from build123d import *

# Parameters (mm, degrees)
CROQUIS1_W              = 633.04
CROQUIS1_H              = 80
CROQUIS1_R              = 4.7625
SALIENTE_EXTRUIR1_DEPTH = 10
CROQUIS2_W              = 633.04
CROQUIS2_H              = 10
SALIENTE_EXTRUIR2_DEPTH = 70
CROQUIS3_R              = 4.7625
CROQUIS3_R_2            = 4.765
CORTAR_EXTRUIR1_DEPTH   = 642.903140357
CORTAR_EXTRUIR2_DEPTH   = 15
CORTAR_EXTRUIR3_DEPTH   = 15


with BuildPart() as part:
    # Croquis1 → Saliente-Extruir1 (new body)
    with BuildSketch(Plane.XY):
        with Locations((316.52, 40)):
            Rectangle(CROQUIS1_W, CROQUIS1_H)
        with Locations((30, 40)):
            Circle(CROQUIS1_R, mode=Mode.SUBTRACT)
        with Locations((603.04, 40)):
            Circle(CROQUIS1_R, mode=Mode.SUBTRACT)
    extrude(amount=SALIENTE_EXTRUIR1_DEPTH)

    # Croquis2 → Saliente-Extruir2 (add)
    with BuildSketch(Plane.XY.offset(10)):
        with Locations((316.52, 75)):
            Rectangle(CROQUIS2_W, CROQUIS2_H)
    extrude(amount=SALIENTE_EXTRUIR2_DEPTH)

    # Croquis3 → Cortar-Extruir1 (cut, through all)
    with BuildSketch(Plane.XZ.offset(-70)):
        with Locations((30, 45)):
            Circle(CROQUIS3_R)
        with Locations((603.04, 45)):
            Circle(CROQUIS3_R_2)
    extrude(amount=-CORTAR_EXTRUIR1_DEPTH, mode=Mode.SUBTRACT)

    # Croquis4 → Cortar-Extruir2 (cut)
    with BuildSketch(Plane(origin=(633.04, 0, 0), x_dir=(0, 0, -1), z_dir=(1, 0, 0))):
        Polygon((-80, 70), (-80, 80), (0, 80), (0, 0), (-10, 0), (-10, 70), align=None)
    extrude(amount=-CORTAR_EXTRUIR2_DEPTH, mode=Mode.SUBTRACT)

    # Croquis5 → Cortar-Extruir3 (cut)
    with BuildSketch(Plane.ZY):
        Polygon((80, 70), (80, 80), (0, 80), (0, 0), (10, 0), (10, 70), align=None)
    extrude(amount=-CORTAR_EXTRUIR3_DEPTH, mode=Mode.SUBTRACT)


solid = part.part
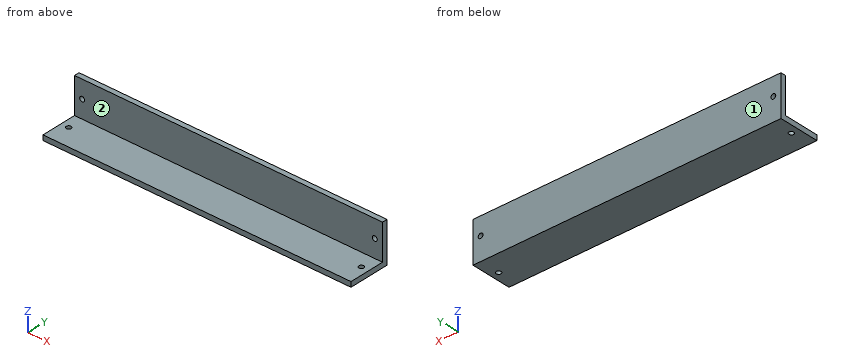
For this review, take the finished solid that the model builds, in its own axes (mm). Face numbers are marked on the shaded views. A direction names the side the tool comes from. Round coordinates to 2 decimals unless told otherwise and drop trailing zeros. Loops run counter-clockwise (first coordinate to the right, second up) from the corner with the lowest first, then second, coordinate; pieces in that order, holes last. Notation, with made-up numbers: (88, -3.75) - (112, -3.75) arc R16 ccw to (112, 4.25) - close; hole circle Ø11 at (19, -35). An arc over 180 degrees is marked (long way). Put each result on its own line as item: value. Start each with the question number.
1. For probe 1 along Y at (x, z) = (30, 5.75); probe 2 along Z at (x, y) = (30, 73); probe 3 along Y at (x, z) = (343.5, 50), list the stretches that pass through material, from the lowest coordinate up. Write a range as [from, to].
2. Consider section C-C on z = 24. State the section outline as (x, y) points, plus the area to 3 significant figures.
3. For the marked faces 1 and 2, list the 3-axis set-ups (+Z, -Z, +X, -X, +Y, -Y) from which the entire face can be reached by the end or side of a thin tool; tool diameter is ignored.
4. Consider section B-B on y = 61.5. State the section outline as (x, z) points.
5. Consider section A-A on x = 167. State the section outline as (y, z) points.
6. Insertion check: P1, Ø15, axis at x = 30, y = 40, coming from the +Z side; P2, Ø3, axis at x = 432.5, z = 17, coming from the -Y side. Each pin has a flat end and moves straight along its axis. Give the tip position at first contact, or say it passes through.
Result sheet:
1. probe 1: [0, 35.24], [44.76, 80]
1. probe 2: [0, 40.24], [49.76, 80]
1. probe 3: [70, 80]
2. outline: (15, 70) - (618.04, 70) - (618.04, 80) - (15, 80) - close
2. area: 6,030 mm^2
3. face 1: +Z, -Z, +X, -X, +Y
3. face 2: +Z, +X, -X, -Y
4. outline: (15, 0) - (618.04, 0) - (618.04, 10) - (15, 10) - close
5. outline: (0, 0) - (80, 0) - (80, 80) - (70, 80) - (70, 10) - (0, 10) - close
6. P1: z = 10
6. P2: y = 70
